The listing builds one solid part. Answer for the finished solid, in the listing's coordinates (mm). A direction names the side the tool comes from. Coordinates: 2 decimals unless noted, no trailing zeros. Order: outer loops, then holes, each group sorted by start corner. A loop starts at its lowest first (then second) coordinate and runs counter-clockwise, first axis right, second up.
Autodesk Inventor part; units mm, degrees
ref_plane "YZ Plane" through (0, 0, 0) normal (1, 0, 0) x (0, 1, 0)
ref_plane "XZ Plane" through (0, 0, 0) normal (0, 1, 0) x (-1, 0, 0)
ref_plane "XY Plane" through (0, 0, 0) normal (0, 0, 1) x (1, 0, 0)
sketch "Sketch1" plane through (0, 0, 0) normal (0, 1, 0) x (-1, 0, 0)
  line L0 (0, 0) -> (61.5, 0)
  line L1 (61.5, 0) -> (61.5, -81.5)
  line L2 (61.5, -81.5) -> (0, -81.5)
  line L3 (0, -81.5) -> (0, 0)
  line L4 (61.5, -40.75) -> (0, -40.75)
  line L5 (30.75, 0) -> (30.75, -81.5)
  line L6 (30.75, -81.5) -> (30.75, 0)
  circle A0 centre (55.65, -6) radius 1.5
  circle A1 centre (5.85, -6) radius 1.5
  circle A2 centre (55.65, -75.5) radius 1.5
  circle A3 centre (5.85, -75.5) radius 1.5
  dimension "d0" = 61.5
  dimension "d1" = 81.5
  dimension "d2" = 69.5
  dimension "d3" = 49.8
  dimension "d4" = 3
extrude "Extrusion1" add sketch "Sketch1" along normal blind 1.5
sketch "Sketch2" plane through (0, 1.5, 0) normal (0, 1, 0) x (1, 0, 0)
  line L0 (-61.5, 81.5) -> (-61.5, 0)
  line L1 (-61.5, 40.75) -> (0, 40.75)
  line L2 (0, 40.75) -> (0, 11.5412)
  line L3 (0, 11.5412) -> (-61.5, 11.5412)
  line L4 (-61.5, 11.5412) -> (-61.5, 40.75)
  line L5 (-61.5, 0) -> (0, 0)
  line L6 (-29.2541, 11.5412) -> (-51.2255, 11.5412)
  line L7 (-61.5, 68.5681) -> (-61.5, 63.2604)
  line L8 (-51.2255, 11.5412) -> (-30.75, 11.5412)
  line L9 (-30.75, 11.5412) -> (-30.75, 0)
  line L10 (-30.75, 0) -> (-51.2255, 0)
  line L11 (-51.2255, 0) -> (-51.2255, 11.5412)
  point P0 (0, 68.5681)
extrude "Extrusion2" add sketch "Sketch2" along normal blind 30 contours L1 L2 L3 L0 | L3 L9 L5 L11
sketch "Sketch3" plane through (0, 0, 0) normal (0, -1, 0) x (1, 0, 0)
  line L0 (-61.5, -81.5) -> (-61.5, 0)
  line L1 (-61.5, -40.75) -> (0, -40.75)
  line L2 (-61.5, -70.6132) -> (0, -70.6132)
  line L3 (0, -70.6132) -> (0, -40.75)
  line L4 (0, -40.75) -> (-61.5, -40.75)
  line L5 (-61.5, -40.75) -> (-61.5, -70.6132)
  line L6 (0, 0) -> (0, -81.5)
  line L7 (-50.2544, -10.7457) -> (0, -10.7457)
  line L8 (0, -10.7457) -> (0, -27.6996)
  line L9 (0, -27.6996) -> (-50.2544, -27.6996)
  line L10 (-50.2544, -27.6996) -> (-50.2544, -10.7457)
extrude "Extrusion3" add sketch "Sketch3" along normal blind 20
properties part number "Platine"
(1) The mould has two halves that part along Z. Classify faces 6 (the face through (-31, -10, -70.613)), 7 (the face through (-25, -10, -27.7)), 8 (the face through (-30, 1.5, -61)): released by +Z, released by -Z, zero draft, split by the parting line, or undercut.
(2) Find section D-D (x = -26.5). Write down the section's boundary in (y, z).
(3) Each of these flat-tipped pins is pushed along its axis until it touches: pin 1 Ø16 at (x, y) = (-25.5, -10.5) entering from -Z; pin 2 Ø10 at (x, y) = (-14, 16.5) entering from -Z; pin 3 Ø5 at (y, z) = (-10.5, -21.5) entering from -X. Where does it stop, or does it pass through?
(4) For faces 1 (the face through (-25, -10, -10.746)), 2 (the face through (-15, 1.5, -6)), 3 (the face through (-50.254, -10, -19)), 4 (the face through (-57.4, 1.5, -5.7)), 5 (the face through (-31, -10, -40.75)), determine the directions among +Z, -Z, +X, -X, +Y, -Y from which every point of the face is accessible in a straight line to the end or side of a thin tool.
(5) Find section A-A (z = -6). Write down the section's boundary in (x, y), and give its area (3 significant figures).
(6) Find section B-B (x = -5.85). Write down the section's boundary in (y, z).
(7) Consider line 1 (Z direction, x = -55.65, y = 0.8); line 2 (X direction, y = 1, z = -75); line 3 (Z direction, x = -38, y = -10.5). Determine where each line is inside the solid, lowest interval first.
(8) Find section C-C (y = -11). Write down the section's boundary in (x, z).
Findings below:
1. face 6: released by -Z
1. face 7: undercut
1. face 8: zero draft
2. outline: (-20, -70.61) - (0, -70.61) - (0, -81.5) - (1.5, -81.5) - (1.5, -40.75) - (31.5, -40.75) - (31.5, -11.54) - (1.5, -11.54) - (1.5, 0) - (0, 0) - (0, -10.75) - (-20, -10.75) - (-20, -27.7) - (0, -27.7) - (0, -40.75) - (-20, -40.75) - close
3. pin 1: stops at z = -70.61
3. pin 2: stops at z = -40.75
3. pin 3: stops at x = -50.25
4. face 1: +Z, +X, -X, -Y
4. face 2: +Z, +X, +Y
4. face 3: +Z, -X, -Y
4. face 4: +Z, -X, +Y
4. face 5: +X, -X, -Y
5. outline: (-61.5, 0) - (-57.15, 0) - (-57.15, 1.5) - (-61.5, 1.5) - close; (-54.15, 0) - (-7.35, 0) - (-7.35, 1.5) - (-30.75, 1.5) - (-30.75, 31.5) - (-51.23, 31.5) - (-51.23, 1.5) - (-54.15, 1.5) - close; (-4.35, 0) - (0, 0) - (0, 1.5) - (-4.35, 1.5) - close
5. area: 698 mm2
6. outline: (-20, -70.61) - (0, -70.61) - (0, -74) - (1.5, -74) - (1.5, -40.75) - (31.5, -40.75) - (31.5, -11.54) - (1.5, -11.54) - (1.5, -7.5) - (0, -7.5) - (0, -10.75) - (-20, -10.75) - (-20, -27.7) - (0, -27.7) - (0, -40.75) - (-20, -40.75) - close; (0, -81.5) - (1.5, -81.5) - (1.5, -77) - (0, -77) - close; (0, -4.5) - (1.5, -4.5) - (1.5, 0) - (0, 0) - close
7. line 1: z = -81.5 to -77, -74 to -7.5, -4.5 to 0
7. line 2: x = -61.5 to -57.06, -54.24 to -7.26, -4.44 to 0
7. line 3: z = -70.61 to -40.75, -27.7 to -10.75
8. outline: (-61.5, -70.61) - (0, -70.61) - (0, -40.75) - (-61.5, -40.75) - close; (-50.25, -27.7) - (0, -27.7) - (0, -10.75) - (-50.25, -10.75) - close
